Part model, mm, in its own coordinate system. Face numbers are marked on the shaded views. A direction names the side the tool comes from. Coordinates: 2 decimals unless noted, no trailing zeros. Loops run counter-clockwise (first coordinate to the right, second up) from the corner with the lowest first, then second, coordinate; pieces in that order, holes last. Notation, with made-up numbers: M -37,18 L 17,18 A36 ccw 17,52 Z; hole C 81,33.5 d11. An arc over 180 degrees is marked long. Use a Markdown table: item, result. Add a question column.
1) Wall check: probe 1 along X at (y, z) = (-50, 24); probe 2 along Z at (x, y) = (-7, 43); probe 3 along Y at (x, z) = (-11, 47). Give the ranges that are in metal, low to high. Write a range as from..to.
2) Tool access for the marked faces 1, 2 and 3: list every direction of +Z, -Z, +X, -X, +Y, -Y with a clear straight run to the whole face (end or side of a thin tool).
3) Pin check, flat tips, straight feed: pin 1 Ø1 at (x, z) = (-10.5, -14.5) entering from -Y; pin 2 Ø3 at (y, z) = (22.5, 66.5) entering from +X; pin 3 Ø4 at (x, y) = (-33.5, -43) entering from -Z. Stop position of each tip, or through.
4) Band-saw the part on A-A (y = -38). List the corners of the cut face in (x, z).
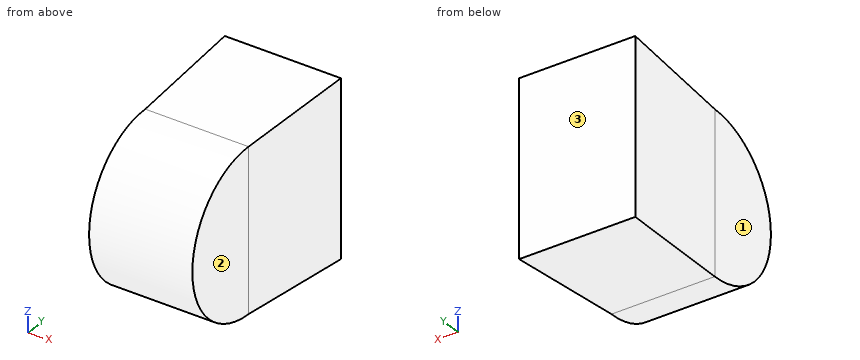
from build123d import *

# Parameters (mm, degrees)
F0_W      = 76.0117769241
F0_H      = 59.1742545366
F1_ANGLE  = 180
F1_FACE_W = 76.0117769241
F1_FACE_H = 118.3485090733
F2_DEPTH  = 90.5473530293
F2_TAPER  = -3


with BuildPart() as f1:
    # F0 (on Front) → F1 (revolve)
    with BuildSketch(Plane.XZ):
        Rectangle(F0_W, F0_H)
    revolve(axis=Axis((0, 0, 29.5871272683), (-1, 0, 0)), revolution_arc=F1_ANGLE)

    # F1_face (on face) → F2 (join)
    with BuildSketch(Plane(origin=(0, 0, 29.5871272683), x_dir=(-1, 0, 0), z_dir=(0, 1, 0))):
        Rectangle(F1_FACE_W, F1_FACE_H)
    extrude(amount=F2_DEPTH, taper=F2_TAPER)


solid = f1.part
Entries:
| question | item | result |
|---|---|---|
| 1 | probe 1 | -38.01..38.01 |
| 1 | probe 2 | -31.84..91.01 |
| 1 | probe 3 | -56.55..90.55 |
| 2 | face 1 | +Z, -Z, -X, -Y |
| 2 | face 2 | +Z, -Z, +X, -Y |
| 2 | face 3 | +Z, -Z, +X, -X, +Y |
| 3 | pin 1 | y = -40.02 |
| 3 | pin 2 | x = 39.26 |
| 3 | pin 3 | z = -13.08 |
| 4 | outline | M -38.01,-15.77 L 38.01,-15.77 L 38.01,74.95 L -38.01,74.95 Z |
